Design review of the part built by this model. Coordinates are the model's own, in mm. Coordinates: 2 decimals unless noted, no trailing zeros. Loops run counter-clockwise (first coordinate to the right, second up) from the corner with the lowest first, then second, coordinate; pieces in that order, holes last. Notation, with made-up numbers: M 8.5,28.5 L 52.5,28.5 A19 cw 52.5,53.5 Z; hole C 42.5,-4 d1. An arc over 180 degrees is marked long. Answer as a JSON object with one key per item and string values. Group by question number.
1. Consider section C-C (y = 67.5). State the section outline as (x, z) points.
2. Insertion check: pin 1 (1.5 mm diameter, centred on x = 168.5, z = 3.5, fed in from +Y); pin 2 (2.5 mm diameter, centred on x = -188.5, z = 3.5, fed in from +Y). Each pin has a flat end and moves straight along its axis. Give the tip position at first contact, or say it passes through.
3. Consider section A-A (z = 3.9). Count the separate pieces of the cut face and the enclosed holes in it, then the cut area to 3 significant figures.
4. Consider section B-B (x = 24). State the section outline as (y, z) points.
5. To check wall thickness, follow probe 1 along X at (y, z) = (10.5, 1.05); probe 2 along Y at (x, z) = (128, 2.45); probe 3 along Y at (x, z) = (208, 3.5). State the ranges of each line that lie inside material, in increasing order.
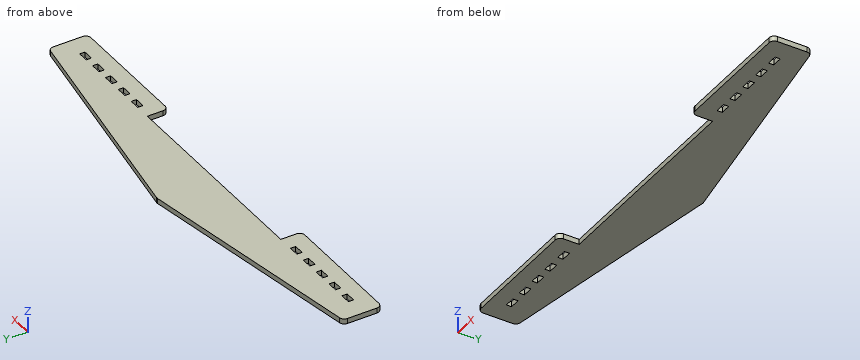
Autodesk Inventor part; units mm, degrees
ref_plane "YZ Plane" through (0, 0, 0) normal (1, 0, 0) x (0, 1, 0)
ref_plane "XZ Plane" through (0, 0, 0) normal (0, 1, 0) x (-1, 0, 0)
ref_plane "XY Plane" through (0, 0, 0) normal (0, 0, 1) x (1, 0, 0)
sketch "Sketch1" plane through (0, 0, 0) normal (0, 0, 1) x (1, 0, 0)
  line L0 (-232.2957, 0) -> (232.2957, 0)
  line L1 (232.2957, 0) -> (232.2957, 38.1)
  line L2 (232.2957, 38.1) -> (-232.2957, 38.1) construction
  line L3 (-232.2957, 38.1) -> (-232.2957, 0)
  line L4 (-232.2957, 38.1) -> (0, 76.2)
  line L5 (0, 76.2) -> (232.2957, 38.1)
  line L6 (0, 76.2) -> (0, 38.1) construction
  point P0 (0, 0)
  point P1 (0, 0)
  dimension "d0" = 464.5914
  dimension "d1" = 38.1
  dimension "d2" = 38.1
extrude "Extrusion1" add sketch "Sketch1" along normal blind 5.08
fillet "Fillet1" radius 5.08 3 edges at (0, 76.2, 2.54) (232.2957, 38.1, 2.54) (-232.2957, 38.1, 2.54)
fillet "Fillet2" radius 5.08 2 edges at (-232.2957, 0, 2.54) (232.2957, 0, 2.54)
sketch "Sketch2" plane through (0, 0, 0) normal (0, 0, -1) x (-1, 0, 0)
  line L0 (-211.9778, 20.32) -> (-201.8178, 20.32)
  line L1 (-201.8178, 20.32) -> (-201.8178, 15.24)
  line L2 (-201.8178, 15.24) -> (-211.9778, 15.24)
  line L3 (-211.9778, 15.24) -> (-211.9778, 20.32)
  line L4 (-191.6578, 20.32) -> (-181.4978, 20.32)
  line L5 (-181.4978, 20.32) -> (-181.4978, 15.24)
  line L6 (-181.4978, 15.24) -> (-191.6578, 15.24)
  line L7 (-191.6578, 15.24) -> (-191.6578, 20.32)
  line L8 (-171.3378, 20.32) -> (-161.1778, 20.32)
  line L9 (-161.1778, 20.32) -> (-161.1778, 15.24)
  line L10 (-161.1778, 15.24) -> (-171.3378, 15.24)
  line L11 (-171.3378, 15.24) -> (-171.3378, 20.32)
  line L12 (-151.0178, 20.32) -> (-140.8578, 20.32)
  line L13 (-140.8578, 20.32) -> (-140.8578, 15.24)
  line L14 (-140.8578, 15.24) -> (-151.0178, 15.24)
  line L15 (-151.0178, 15.24) -> (-151.0178, 20.32)
  line L16 (-130.6978, 20.32) -> (-120.5378, 20.32)
  line L17 (-120.5378, 20.32) -> (-120.5378, 15.24)
  line L18 (-120.5378, 15.24) -> (-130.6978, 15.24)
  line L19 (-130.6978, 15.24) -> (-130.6978, 20.32)
  line L20 (-45.72, 20.32) -> (-45.72, 15.24)
  line L21 (-45.72, 15.24) -> (-105.2978, 15.24) construction
  line L22 (-105.2978, 15.24) -> (-105.2978, 20.32)
  line L23 (-105.2978, 20.32) -> (-45.72, 20.32)
  line L24 (-40.64, 15.24) -> (-40.64, 20.32)
  line L25 (-40.64, 20.32) -> (40.64, 20.32)
  line L26 (40.64, 20.32) -> (40.64, 15.24)
  line L27 (40.64, 15.24) -> (-40.64, 15.24) construction
  line L28 (45.72, 15.24) -> (45.72, 20.32)
  line L29 (45.72, 20.32) -> (105.2978, 20.32)
  line L30 (105.2978, 20.32) -> (105.2978, 15.24)
  line L31 (105.2978, 15.24) -> (45.72, 15.24) construction
  arc A0 (-232.2957, 5.08) -> (-227.2157, 0) centre (-227.2157, 5.08) ccw
  line L32 (227.2157, 0) -> (-227.2157, 0)
  arc A1 (227.2157, 0) -> (232.2957, 5.08) centre (227.2157, 5.08) ccw
  line L33 (232.2957, 33.7853) -> (232.2957, 5.08)
  arc A2 (232.2957, 33.7853) -> (228.0379, 38.7983) centre (227.2157, 33.7853) ccw
  line L34 (0.8222, 76.0651) -> (228.0379, 38.7983) construction
  arc A3 (0.8222, 76.0651) -> (-0.8222, 76.0651) centre (0, 71.0521) ccw construction
  line L35 (-228.0379, 38.7983) -> (-0.8222, 76.0651) construction
  arc A4 (-228.0379, 38.7983) -> (-232.2957, 33.7853) centre (-227.2157, 33.7853) ccw
  line L36 (-232.2957, 5.08) -> (-232.2957, 33.7853)
  line L37 (-105.2978, 15.24) -> (-105.2978, 0)
  line L38 (227.2157, 0) -> (-227.2157, 0)
  line L39 (-105.2978, 20.32) -> (105.2978, 20.32)
  line L40 (105.2978, 20.32) -> (105.2978, 0)
  line L41 (105.2978, 0) -> (-105.2978, 0)
  line L42 (-105.2978, 0) -> (-105.2978, 20.32)
  point P0 (0, 0)
extrude "Extrusion2" cut sketch "Sketch2" against normal blind 5.08
fillet "Fillet3" radius 5.08 2 edges at (105.2978, 0, 2.54) (-105.2978, 0, 2.54)
mirror "Mirror1" about plane through (0, 0, 0) normal (1, 0, 0) of "Extrusion2"
properties part number "TrusSupport" material "Wood (Birch)"
Findings below:
{
 "1": {"outline": "M -53.04,0 L 53.04,0 L 53.04,5.08 L -53.04,5.08 Z"},
 "2": {"pin 1": "stops at y = 48.69", "pin 2": "stops at y = 45.49"},
 "3": {"separate pieces": "1", "enclosed holes": "10", "area": "21,700 mm^2"},
 "4": {"outline": "M 20.32,0 L 72.26,0 L 72.26,5.08 L 20.32,5.08 Z"},
 "5": {"probe 1": "x = -232.3 to -105.3, 105.3 to 232.3", "probe 2": "y = 0 to 15.24, 20.32 to 55.21", "probe 3": "y = 0 to 15.24, 20.32 to 42.08"}
}
